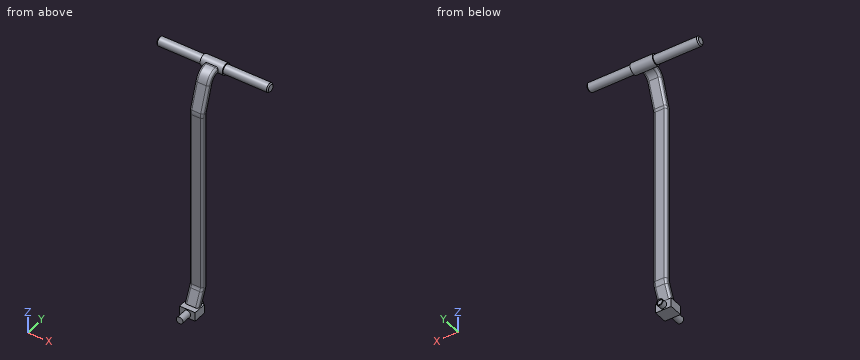
from build123d import *

# Parameters (mm, degrees)
F3_R      = 25
F4_DEPTH  = 50
F5_R      = 20
F6_DEPTH  = 250
F7_SIZE   = 5
F8_W      = 60
F8_H      = 40
F9_DEPTH  = 35
F10_R     = 15
F11_DEPTH = 25
F12_R     = 15
F13_DEPTH = 50
F14_R     = 12.5
F15_DEPTH = 5
F16_R     = 2


with BuildPart() as f2:
    # F2: sweep along a path in F1
    with BuildLine(Plane.YZ) as f2_path:
        Line((0, 0), (35.6326628073, 79.5632662807))
        ThreePointArc((35.6326628073, 79.5632662807), (38.8959770348, 89.5509124888), (40, 100))
        Line((40, 100), (40, 500))
        Line((40, 500), (40, 891.8861169916))
        ThreePointArc((40, 891.8861169916), (40.6456271181, 899.8952291419), (42.5658350975, 907.6975052924))
        Line((42.5658350975, 907.6975052924), (78.6037961003, 1015.8113883008))
        ThreePointArc((78.6037961003, 1015.8113883008), (96.8024467696, 1040.5621092588), (126.0379610028, 1050))
        Line((126.0379610028, 1050), (150, 1050))
    # F0 (on Top) → F2 (sweep)
    with BuildSketch(Plane.XY):
        with BuildLine():
            Line((-20, -15), (20, -15))
            ThreePointArc((20, -15), (27.0710678119, -12.0710678119), (30, -5))
            Line((30, -5), (30, 5))
            ThreePointArc((30, 5), (27.0710678119, 12.0710678119), (20, 15))
            Line((20, 15), (-20, 15))
            ThreePointArc((-20, 15), (-27.0710678119, 12.0710678119), (-30, 5))
            Line((-30, 5), (-30, -5))
            ThreePointArc((-30, -5), (-27.0710678119, -12.0710678119), (-20, -15))
        make_face()
        with BuildLine():
            Line((-20, 10), (20, 10))
            ThreePointArc((20, 10), (23.5355339059, 8.5355339059), (25, 5))
            Line((25, 5), (25, -5))
            ThreePointArc((25, -5), (23.5355339059, -8.5355339059), (20, -10))
            Line((20, -10), (-20, -10))
            ThreePointArc((-20, -10), (-23.5355339059, -8.5355339059), (-25, -5))
            Line((-25, -5), (-25, 5))
            ThreePointArc((-25, 5), (-23.5355339059, 8.5355339059), (-20, 10))
        make_face(mode=Mode.SUBTRACT)
    sweep(path=f2_path.line)

    # F3 (on Right) → F4 (join, symmetric)
    with BuildSketch(Plane.YZ):
        with Locations((149.1591930389, 1051.1897988422)):
            Circle(F3_R)
    extrude(amount=F4_DEPTH, both=True)

    # F5 (on Right) → F6 (join, symmetric)
    with BuildSketch(Plane.YZ):
        with Locations((149.1591930389, 1051.1897988422)):
            Circle(F5_R)
    extrude(amount=F6_DEPTH, both=True)

    # F7
    f7_edges = [f2.edges().sort_by_distance(p)[0] for p in [
        (-250, 129.159193, 1051.189799),
        (250, 129.159193, 1051.189799),
    ]]
    chamfer(f7_edges, length=F7_SIZE)

    # F8 (on Right) → F9 (join, symmetric)
    with BuildSketch(Plane.YZ):
        Rectangle(F8_W, F8_H)
    extrude(amount=F9_DEPTH, both=True)

    # F10 (on face) → F11 (join)
    with BuildSketch(Plane(origin=(0, 30, 0), x_dir=(-1, 0, 0), z_dir=(0, 1, 0))):
        Circle(F10_R)
    extrude(amount=F11_DEPTH)

    # F12 (on face) → F13 (join)
    with BuildSketch(Plane.XZ.offset(30)):
        Circle(F12_R)
    extrude(amount=F13_DEPTH)

    # F14 (on face) → F15 (cut)
    with BuildSketch(Plane(origin=(0, 55, 0), x_dir=(-1, 0, 0), z_dir=(0, 1, 0))):
        Circle(F14_R)
    extrude(amount=-F15_DEPTH, mode=Mode.SUBTRACT)

    # F16
    f16_edges = [f2.edges().sort_by_distance(p)[0] for p in [
        (15, 55, 0),
    ]]
    fillet(f16_edges, radius=F16_R)


solid = f2.part
Can you work these out from the model? Positions are in its coordinate system, mm. Give positions to 0.01 mm unless a question says otherwise; leave off trailing zeros. Order: outer loops, then holes, each group sorted by start corner. A loop starts at its lowest first (then second) coordinate and runs counter-clockwise, first axis right, second up. Notation, with made-up numbers: (61, 6.25) - (93, 6.25) arc R19 cw to (93, 42.25) - close; hole circle Ø1 at (6.5, -32.5). An arc over 180 degrees is marked (long way). Write each question's results on one line, items separated by ' | '.
1) Suppose I cut it at A-A, the plane z = 0. Write out the boundary of the cut face in (x, y).
Final values:
outline: (-35, -30) - (-15, -30) - (-15, -80) - (15, -80) - (15, -30) - (35, -30) - (35, 30) - (15, 30) - (15, 53) arc R2 ccw to (13, 55) - (12.5, 55) - (12.5, 50) - (-12.5, 50) - (-12.5, 55) - (-13, 55) arc R2 ccw to (-15, 53) - (-15, 30) - (-35, 30) - close
2) Suppose I cut it at B-B, the plane y = -18. Write out the boundary of the cut face in (x, z), then the cut area to 3 significant figures.
Final values:
outline: (-35, -20) - (35, -20) - (35, 20) - (-35, 20) - close | area: 2,800 mm^2
3) Suppose I cut it at C-C, the plane x = 196.5. Write out the boundary of the cut face in (y, z).
Final values:
outline: circle Ø40 at (149.16, 1051.19)
4) I'm going to push flat-ended pins straight in: pin 1 Ø5 at (y, z) = (46, 649) entering from +X; pin 2 Ø2.5 at (x, y) = (-2.5, 124.5) entering from +Z; pin 3 Ø18 at (x, y) = (-17.5, 3) entering from +Z. Where does each tip first touch, or does it pass through?
Final values:
pin 1: stops at x = 30 | pin 2: stops at z = 1063.69 | pin 3: stops at z = 60.29
5) Please list where these lines run through material, in increasing order: line 1 along Y through (x, z) = (15, 743.5); line 2 along X through (y, z) = (86.5, 1023); line 3 along Z through (x, y) = (-96, 142). Write a range as [from, to].
Final values:
line 1: y = [26.31, 30.87], [49.13, 53.69] | line 2: x = [-30, -25], [25, 30] | line 3: z = [1032.52, 1069.86]
